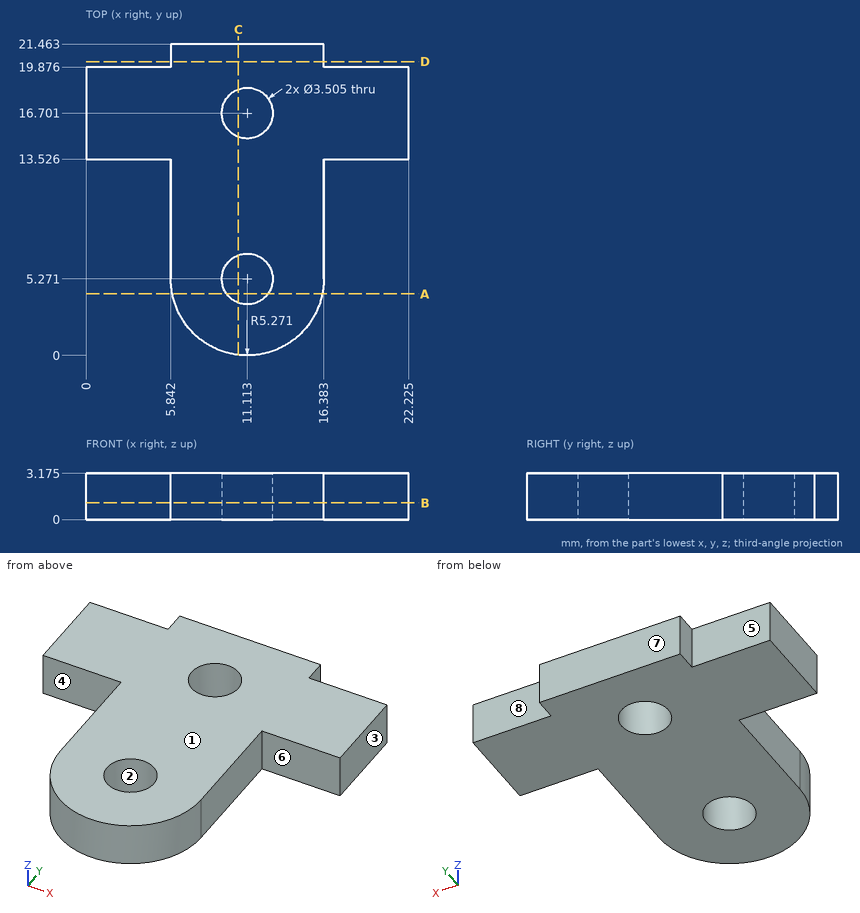
Design review of the part shown in the three views and the two pictorial views. Dimensions are in mm from the part's minimum x, y and z. A direction names the side the tool comes from. Round coordinates to 2 decimals unless told otherwise and drop trailing zeros. Loops run counter-clockwise (first coordinate to the right, second up) from the corner with the lowest first, then second, coordinate; pieces in that order, holes last.
(1) Wall thickness on line 1 along Y through (x, z) = (10, 3) (1 decimal); line 2 along Y through (x, z) = (11.75, 1.55); line 3 along X through (y, z) = (12, 1.8): over which ranges is each line inside the solid? List them lowest first.
Returned:
line 1: y = 0.1 to 3.9, 6.6 to 15.3, 18.1 to 21.5
line 2: y = 0.04 to 3.64, 6.9 to 15.07, 18.33 to 21.46
line 3: x = 5.84 to 16.38
(2) Mouldability with a two-part tool opening along X and no side actions: class the marked faces 1, 2 and 3 as released by +X, released by -X, zero draft, split by the parting line, or undercut.
Returned:
face 1: zero draft
face 2: undercut
face 3: released by +X
(3) We need section B-B (z = 1.15). Give the boundary of the cut face in (x, y) (1 decimal).
Returned:
outline: (0, 13.5) - (5.8, 13.5) - (5.8, 5.3) arc R5.3 ccw to (16.4, 5.3) - (16.4, 13.5) - (22.2, 13.5) - (22.2, 19.9) - (16.4, 19.9) - (16.4, 21.5) - (5.8, 21.5) - (5.8, 19.9) - (0, 19.9) - close; hole circle Ø3.5 at (11.1, 5.3); hole circle Ø3.5 at (11.1, 16.7)
(4) Tool access review of the marked faces 4, 5, 6, 7 and 8: name each direction out of +Z, -Z, +X, -X, +Y, -Y from which nothing blocks a thin tool from reaching the whole face with its end or side.
Returned:
face 4: +Z, -Z, -X, -Y
face 5: +Z, -Z, -X, +Y
face 6: +Z, -Z, +X, -Y
face 7: +Z, -Z, +X, -X, +Y
face 8: +Z, -Z, +X, +Y
(5) We need section C-C (x = 10.5). Give the boundary of the cut face in (y, z) (1 decimal).
Returned:
outline: (0, 0) - (3.6, 0) - (3.6, 3.2) - (0, 3.2) - close; (6.9, 0) - (15.1, 0) - (15.1, 3.2) - (6.9, 3.2) - close; (18.3, 0) - (21.5, 0) - (21.5, 3.2) - (18.3, 3.2) - close
(6) Clearance check with flat-ended pins moving along their axes: P1, Ø3, axis at x = 11.11, y = 16.7, coming from the -Z side; P2, Ø0.8, axis at y = 20.5, z = 1, coming from the +X side; P3, Ø1, axis at x = 4, z = 1.5, coming from the -Y side (1 decimal); P4, Ø1, axis at x = 1.5, z = 1, coming from the +Y side (1 decimal). State where each tip first meets the part, or that it passes through.
Returned:
P1: passes through
P2: stops at x = 16.38
P3: stops at y = 13.5
P4: stops at y = 19.9
(7) We need section A-A (y = 4.25). Give the boundary of the cut face in (x, z) (1 decimal).
Returned:
outline: (5.9, 0) - (9.7, 0) - (9.7, 3.2) - (5.9, 3.2) - close; (12.5, 0) - (16.3, 0) - (16.3, 3.2) - (12.5, 3.2) - close
(8) We need section D-D (y = 20.25). Give the boundary of the cut face in (x, z) (1 decimal).
Returned:
outline: (5.8, 0) - (16.4, 0) - (16.4, 3.2) - (5.8, 3.2) - close
